Read the model definition and answer for the solid it produces. Units are mm, in the model's axes. A direction names the side the tool comes from. Coordinates: 2 decimals unless noted, no trailing zeros. Loops run counter-clockwise (first coordinate to the right, second up) from the corner with the lowest first, then second, coordinate; pieces in that order, holes last. Notation, with made-up numbers: (62.25, 40) - (79.25, 40) arc R13 cw to (79.25, 64) - close; hole circle Ø7 at (-5, 19). An arc over 180 degrees is marked (long way). Use one line per item in the form item = value. Start each with the question number.
1) A cutting plane is placed at B-B (x = 132). Give the vertices of the cut face in (y, z), and give its area (3 significant figures).
2) A cutting plane is placed at A-A (y = 22). State how many separate pieces and enclosed holes the cut face has, and give its area (3 significant figures).
3) Each of these flat-tipped pins is pushed along its axis until it touches: P1, Ø1.5, axis at x = 76.5, z = -231.5, coming from the +Y side; P2, Ø3, axis at y = 41, z = -97, coming from the +X side; P3, Ø6, axis at y = 45.5, z = -56.5, coming from the +X side. Where does it stop, or does it pass through?
4) A cutting plane is placed at C-C (z = 112.5). Give the vertices of the cut face in (x, y), and give its area (3 significant figures).
5) The mould has two halves that part along Z. Classify faces 3 (the face through (224.53, 48.66, 49.86)), 4 (the face through (249, 38, 55)), 5 (the face through (-229.094, 39.676, -1.432)), 6 (the face through (-4.4, 14.606, 4.4)): released by +Z, released by -Z, zero draft, split by the parting line, or undercut.
6) Consider line 1 (X direction, y = 41, z = 0); line 2 (X direction, y = 32.5, z = -101.5); line 3 (X direction, y = 40.5, z = 101). Determine where each line is inside the solid, lowest interval first.
7) Which of the six approach directions +Z, -Z, +X, -X, +Y, -Y give full straight-line access (tool end or side, diameter ignored) to faces 1 (the face through (-3, 52.606, -48)), 2 (the face through (37, 44.606, 228))?
from build123d import *

# Parameters (mm, degrees)
SKETCH2_R               = 11
CUT_EXTRUDE1_DEPTH      = 10
SKETCH3_R               = 6
CUT_EXTRUDE2_DEPTH      = 447.486281987
CUT_EXTRUDE3_DEPTH      = 88
CUT_EXTRUDE3_DEPTH_BACK = 69
SKETCH4_R               = 6


with BuildPart() as part:
    # Sketch1 → Revolve1 (revolve)
    with BuildSketch(Plane(origin=(0, 0, 0), x_dir=(0, 0, -1), z_dir=(1, 0, 0)), mode=Mode.PRIVATE) as revolve1_sk:
        Polygon((-315.000000002, 14.605962764), (-315.000000002, 44.605962764), (-295.000000002, 44.605962764), (-295.000000002, 31.605962764), (-255.000000002, 31.605962764), (-255.000000002, 44.605962764), (-230, 44.605962764), (-230, 52.605962764), (0, 52.605962764), (0, 44.605962764), (0, 14.605962764), (-229.500000002, 14.605962764), align=None)
    revolve(revolve1_sk.sketch.rotate(Axis((0, -1000, 0), (0, 1, 0)), 180), axis=Axis((0, -1000, 0), (0, 1, 0)))

    # Sketch2 → Cut-Extrude1 (cut)
    with BuildSketch(Plane(origin=(0, 44.605962764, 0), x_dir=(1, 0, 0), z_dir=(0, 1, 0))):
        with Locations(Location((0, 240, 0), (0, 0, 270))):
            Circle(SKETCH2_R)
        with Locations(Location((169.705627485, 169.705627485, 0), (0, 0, 270))):
            Circle(SKETCH2_R)
        with Locations(Location((240, 0, 0), (0, 0, 270))):
            Circle(SKETCH2_R)
        with Locations(Location((169.705627485, -169.705627485, 0), (0, 0, 270))):
            Circle(SKETCH2_R)
        with Locations(Location((0, -240, 0), (0, 0, 270))):
            Circle(SKETCH2_R)
        with Locations(Location((-169.705627485, -169.705627485, 0), (0, 0, 270))):
            Circle(SKETCH2_R)
        with Locations(Location((-240, 0, 0), (0, 0, 270))):
            Circle(SKETCH2_R)
        with Locations(Location((-169.705627485, 169.705627485, 0), (0, 0, 270))):
            Circle(SKETCH2_R)
    extrude(amount=-CUT_EXTRUDE1_DEPTH, mode=Mode.SUBTRACT)

    # Sketch3 → Cut-Extrude2 (cut, through all)
    with BuildSketch(Plane(origin=(0, 44.605962764, 0), x_dir=(1, 0, 0), z_dir=(0, 1, 0))):
        with Locations(Location((0, 240, 0), (0, 0, 270))):
            Circle(SKETCH3_R)
        with Locations(Location((169.705627485, 169.705627485, 0), (0, 0, 270))):
            Circle(SKETCH3_R)
        with Locations(Location((240, 0, 0), (0, 0, 270))):
            Circle(SKETCH3_R)
        with Locations(Location((169.705627485, -169.705627485, 0), (0, 0, 270))):
            Circle(SKETCH3_R)
        with Locations(Location((0, -240, 0), (0, 0, 270))):
            Circle(SKETCH3_R)
        with Locations(Location((-169.705627485, -169.705627485, 0), (0, 0, 270))):
            Circle(SKETCH3_R)
        with Locations(Location((-240, 0, 0), (0, 0, 270))):
            Circle(SKETCH3_R)
        with Locations(Location((-169.705627485, 169.705627485, 0), (0, 0, 270))):
            Circle(SKETCH3_R)
    extrude(amount=-CUT_EXTRUDE2_DEPTH, mode=Mode.SUBTRACT)

    # Sketch4 → Cut-Extrude3 (cut, two sides: drawn at the far end of the back side and taken through both)
    with BuildSketch(Plane(origin=(0, 14.605962764, 0), x_dir=(1, 0, 0), z_dir=(0, 1, 0)).offset(-CUT_EXTRUDE3_DEPTH_BACK)):
        with Locations(Location((0, 0, 0), (0, 0, 90))):
            Circle(SKETCH4_R)
    extrude(amount=CUT_EXTRUDE3_DEPTH + CUT_EXTRUDE3_DEPTH_BACK, mode=Mode.SUBTRACT)


solid = part.part
Found:
q1.outline = (14.61, -286.01) - (44.61, -286.01) - (44.61, -263.82) - (31.61, -263.82) - (31.61, -218.18) - (44.61, -218.18) - (44.61, -188.35) - (52.61, -188.35) - (52.61, 188.35) - (44.61, 188.35) - (44.61, 218.18) - (31.61, 218.18) - (31.61, 263.82) - (44.61, 263.82) - (44.61, 286.01) - (14.61, 286.01) - close
q1.area = 19,000 mm^2
q2.separate_pieces = 1
q2.enclosed_holes = 9
q2.area = 311,000 mm^2
q3.P1 = 44.61
q3.P2 = 300.17
q3.P3 = 310.4
q4.outline = (-294.23, 14.61) - (294.23, 14.61) - (294.23, 44.61) - (272.71, 44.61) - (272.71, 31.61) - (228.84, 31.61) - (228.84, 44.61) - (200.61, 44.61) - (200.61, 52.61) - (-200.61, 52.61) - (-200.61, 44.61) - (-228.84, 44.61) - (-228.84, 31.61) - (-272.71, 31.61) - (-272.71, 44.61) - (-294.23, 44.61) - close
q4.area = 19,700 mm^2
q5.face_3 = split by the parting line
q5.face_4 = undercut
q5.face_5 = undercut
q5.face_6 = zero draft
q6.line_1 = -315 to -295, -255 to -251, -229 to -6, 6 to 229, 251 to 255, 295 to 315
q6.line_2 = -298.2 to -276.99, -233.93 to 233.93, 276.99 to 298.2
q6.line_3 = -298.37 to -277.17, -234.15 to 234.15, 277.17 to 298.37
q7.face_1 = +Z, -Z, +X, -X, +Y
q7.face_2 = +Y
